```python
from build123d import *

# Parameters (mm, degrees)
F1_DEPTH = 20
F2_W     = 20
F2_H     = 2
F3_DEPTH = 12.5
F4_R     = 1


with BuildPart() as f1:
    # F0 (on Front) → F1 (new body)
    with BuildSketch(Plane.XZ):
        Polygon((-10, -7.265425), (-10, -30.776835), (3.81966, -11.755705), (26.18034, -19.02113), (12.36068, 0), (26.18034, 19.02113), (3.81966, 11.755705), (-10, 30.776835), (-10, 7.265425), (-32.36068, 0), align=None)
    extrude(amount=F1_DEPTH)

    # F2 (on Top) → F3 (cut, symmetric)
    with BuildSketch(Plane.XY):
        with Locations((-22.36068, -10)):
            Rectangle(F2_W, F2_H)
    extrude(amount=F3_DEPTH, both=True, mode=Mode.SUBTRACT)

    # F4
    f4_edges = [f1.edges().sort_by_distance(p)[0] for p in [
        (-21.18034, 0, -3.632713),
        (-21.18034, 0, 3.632713),
        (-10, 0, 19.02113),
        (-3.09017, 0, 21.26627),
        (15, 0, 15.388418),
        (19.27051, 0, 9.510565),
        (19.27051, 0, -9.510565),
        (15, 0, -15.388418),
        (-3.09017, 0, -21.26627),
        (-10, 0, -19.02113),
        (-21.18034, -20, 3.632713),
        (-21.18034, -20, -3.632713),
        (-10, -20, -19.02113),
        (-3.09017, -20, -21.26627),
        (15, -20, -15.388418),
        (19.27051, -20, -9.510565),
        (19.27051, -20, 9.510565),
        (15, -20, 15.388418),
        (-3.09017, -20, 21.26627),
        (-10, -20, 19.02113),
        (-10, -10, -30.776835),
        (3.81966, -10, -11.755705),
        (-32.36068, -15.5, 0),
        (-32.36068, -4.5, 0),
        (-10, -10, 30.776835),
        (26.18034, -10, 19.02113),
        (26.18034, -10, -19.02113),
    ]]
    fillet(f4_edges, radius=F4_R)


solid = f1.part
```
Can you work these out from the model? Positions are in its coordinate system, mm. A direction names the side the tool comes from. Give positions to 0.01 mm unless a question says otherwise; leave off trailing zeros. Loops run counter-clockwise (first coordinate to the right, second up) from the corner with the lowest first, then second, coordinate; pieces in that order, holes last. Notation, with made-up numbers: M 82.5,-27.75 L 104.5,-27.75 A4 ccw 104.5,-23.75 Z; hole C 35,-8.75 d9. An arc over 180 degrees is marked long. One line per question, with ' | ' between items. Start each with the question number.
Q1. If we mould it in two halves opening along Z, with no side actions, what happens to faces 1 (the flat face through (1, 0, 2)), 2 (the cylindrical face through (17.822, -19.715, -8.029)), 3 (the cylindrical face through (-9.326, -10.126, -28.645)), 4 (the cylindrical face through (24.382, -10.126, 17.692))? For each: +Z half, -Z half, draft (parallel to the pull), parting line (faces both ways), or undercut.
Q2. If we section it at A-A (y = -12.75): Please give me the cut outline in (x, z).
Q3. For pin 1 Ø4 at (x, y) = (-22, -12.5) entering from +Z; pin 2 Ø0.6 at (y, z) = (-10, 3) entering from -X; pin 3 Ø6 at (y, z) = (-15, 19.5) entering from -X, each with a flat end and sliding along its axis, tell me the tip position at first contact or that it passes through.
Q4. For faces 5 (the cylindrical face through (13.143, -19.715, 14.469)), 6 (the cylindrical face through (13.143, -0.285, 14.469)), 7 (the flat face through (-12.361, -10, 0)), which set-ups out of +Z, -Z, +X, -X, +Y, -Y let a thin tool reach every point of the face, with its end or its side?
Q5. If I drill on line 1 (Z direction, x = 20, y = -8.25); line 2 (Z direction, x = 13, y = -14.25); line 3 (X direction, y = -9.5, z = 25), over which ranges is the centre line in solid material (lowest first)? Write a range as from..to.
Computed:
1) face 1: draft | face 2: undercut | face 3: -Z half | face 4: undercut
2) outline: M -29.43,-0.95 L -10,-7.27 L -10,-27.7 A1 ccw -8.19,-28.29 L 3.39,-12.34 A1 cw 4.51,-11.98 L 23.25,-18.07 A1 ccw 24.37,-16.53 L 12.36,0 L 24.37,16.53 A1 ccw 23.25,18.07 L 3.82,11.76 L -8.19,28.29 A1 ccw -10,27.7 L -10,7.27 L -29.43,0.95 A1 ccw Z
3) pin 1: stops at z = 4.02 | pin 2: stops at x = -12.36 | pin 3: stops at x = -10
4) face 5: +Z, -Y | face 6: +Z, +Y | face 7: +Z, -Z, -X
5) line 1: z = -17.01..-10.51, 10.51..17.01 | line 2: z = -14.74..-0.88, 0.88..14.74 | line 3: x = -10..-5.8
